Could you check a few things on this model? Use its own coordinates, in mm. A direction names the side the tool comes from. Round coordinates to 2 decimals unless told otherwise and drop trailing zeros. Order: outer loops, then holes, each group sorted by start corner. A loop starts at its lowest first (then second) coordinate and runs counter-clockwise, first axis right, second up. Notation, with made-up numbers: (60.5, 56.25) -> (73.5, 56.25) arc R23 ccw to (73.5, 86.25) -> close; hole circle Ø9 at (74, -2.5). An arc over 180 degrees is marked (long way). Put each result on its own line as item: value. Start each with the question number.
from build123d import *

# Parameters (mm, degrees)
F0_W      = 20
F0_H      = 40
F1_DEPTH  = 20
F3_D      = 12
F5_D      = 4.2
F5_DEPTH  = 5
F5_TIP    = 1.2618073
F8_SIZE   = 1
F9_W      = 26
F9_H      = 16
F10_DEPTH = 10
F12_D     = 4.2


# Not quite as in the source:
# - a feature of the source that left no trace in its solid (it failed there, or was rolled back) is left out


with BuildPart() as f1:
    # F0 (on Top) → F1 (new body)
    with BuildSketch(Plane.XY):
        with Locations((10, 20)):
            Rectangle(F0_W, F0_H)
    extrude(amount=F1_DEPTH)

    # F3 (through all)
    with Locations(Plane.XY.offset(20)):
        with Locations((10, 20)):
            Hole(F3_D / 2)

    # F5
    with Locations(Plane(origin=(0, 0, 0), x_dir=(0, -1, 0), z_dir=(-1, 0, 0))):
        with Locations((-20, 10)):
            Hole(F5_D / 2, depth=F5_DEPTH)
            with Locations((0, 0, -(F5_DEPTH + F5_TIP / 2))):  # 118° drill point
                Cone(0, F5_D / 2, F5_TIP, mode=Mode.SUBTRACT)

    # F8
    f8_edges = [f1.edges().sort_by_distance(p)[0] for p in [
        (10, 0, 20),
        (0, 20, 20),
        (10, 40, 20),
    ]]
    chamfer(f8_edges, length=F8_SIZE)

    # F9 (on face) → F10 (join)
    with BuildSketch(Plane.YZ.offset(20)):
        with Locations((20, 10)):
            Rectangle(F9_W, F9_H)
    extrude(amount=F10_DEPTH)

    # F12 (through all)
    with Locations(Plane.XZ.offset(-7)):
        with Locations((25, 10)):
            Hole(F12_D / 2)


solid = f1.part
1. If we section it at D-D, the plane z = 10: Please give me the cut outline in (x, y), then the cut area to 3 significant figures.
2. Which directions (+Z, -Z, +X, -X, +Y, -Y) give clear straight access to the entire face, cutting with the end or side of a thin tool? Please do faces 5 (the face through (25, 20, 2)), 6 (the face through (2.22, 17.9, 10.09)), 7 (the face through (25, 20, 18)), 8 (the face through (22.7, 7, 9.9)), 9 (the face through (22.7, 33, 9.9)).
3. I need wall thicknesses on L1, parallel to Z at x = 3.05, y = 20; L2, parallel to Z at x = 25, y = 14.25; L3, parallel to Y at x = 1, z = 10. Which ranges of each line are inside material? Lowest first, please.
4. For pin 1 Ø5 at (x, y) = (9.5, 34) entering from -Z; pin 2 Ø8 at (x, y) = (27, 16) entering from +Z; pin 3 Ø11 at (x, y) = (26, 18.5) entering from -Z; pin 4 Ø3 at (x, z) = (27, 6.5) entering from +Y, each with a flat end and sliding along its axis, tell me the tip position at first contact or that it passes through.
5. Thinking about a two-plate mould opening in X: for faces 1 (the face through (10, 0, 9)), 2 (the face through (14.76, 16.35, 9.86)), 3 (the face through (25.273, 20.182, 12.082)), 4 (the face through (0.5, 19.7, 19.5)), which applies, +X half, -X half, draft (parallel to the pull), parting line (faces both ways), or undercut?
6. If we section it at C-C, the plane y = 31: Please give me the cut outline in (x, z), then the cut area to 3 significant figures.
7. If we section it at A-A, the plane y = 20: Please give me the cut outline in (x, z).
8. If we section it at B-B, the plane x = 10: Please give me the cut outline in (y, z).
Results below:
1. outline: (0, 0) -> (20, 0) -> (20, 7) -> (22.9, 7) -> (22.9, 33) -> (20, 33) -> (20, 40) -> (0, 40) -> (0, 22.1) -> (4.38, 22.1) arc R6 cw (long way) to (4.38, 17.9) -> (0, 17.9) -> close; (27.1, 7) -> (30, 7) -> (30, 33) -> (27.1, 33) -> close
1. area: 820 mm2
2. face 5: -Z, +X, +Y, -Y
2. face 6: -X
2. face 7: +Z, +X, +Y, -Y
2. face 8: +Z, -Z, +X, -Y
2. face 9: +Z, -Z, +X, +Y
3. L1: 0 to 7.9, 12.1 to 20
3. L2: 2 to 7.9, 12.1 to 18
3. L3: 0 to 17.9, 22.1 to 40
4. pin 1: z = 0
4. pin 2: z = 18
4. pin 3: z = 2
4. pin 4: y = 33
5. face 1: draft
5. face 2: undercut
5. face 3: undercut
5. face 4: -X half
6. outline: (0, 0) -> (20, 0) -> (20, 2) -> (30, 2) -> (30, 18) -> (20, 18) -> (20, 20) -> (1, 20) -> (0, 19) -> close; hole circle Ø4.2 at (25, 10)
6. area: 546 mm2
7. outline: (0, 0) -> (4, 0) -> (4, 7.9) -> (0, 7.9) -> close; (0, 12.1) -> (4, 12.1) -> (4, 20) -> (1, 20) -> (0, 19) -> close; (16, 0) -> (20, 0) -> (20, 2) -> (30, 2) -> (30, 18) -> (20, 18) -> (20, 20) -> (16, 20) -> close; hole circle Ø4.2 at (25, 10)
8. outline: (0, 0) -> (14, 0) -> (14, 20) -> (1, 20) -> (0, 19) -> close; (26, 0) -> (40, 0) -> (40, 19) -> (39, 20) -> (26, 20) -> close
